Input: dimensioned drawing with shaded views. Units: mm. Origin: part minimum x, y, z. A direction names the side the tool comes from. Give positions to 0.01 mm unless a question says otherwise; leave off trailing zeros. Write each loop counter-clockwise with the first axis right and the second up, starting at its lowest first coordinate (ties: lowest second). Pieces come first, ordered by that corner, then holes.
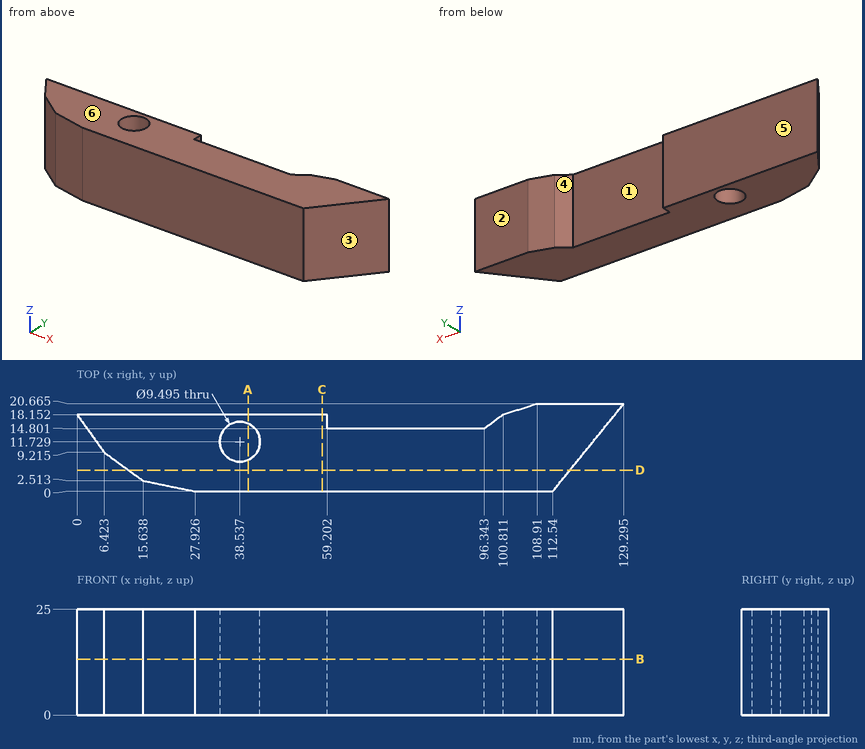
Item 1: Pull-direction query (X, two-part tool) for the marked faces 1, 2 and 3; classes: +X half, -X half, draft (parallel to the pull), parting line (faces both ways), or undercut.
Found:
face 1: undercut
face 2: draft
face 3: +X half
Item 2: Section D-D, the plane y = 5. Return the cut outline in (x, z), plus the area to 3 significant figures.
Found:
outline: (12.22, 0) - (116.59, 0) - (116.59, 25) - (12.22, 25) - close
area: 2,610 mm2
Item 3: Section B-B, the plane z = 13.25. Return the cut outline in (x, y) (1 decimal).
Found:
outline: (0, 18.2) - (6.4, 9.2) - (15.6, 2.5) - (27.9, 0) - (112.5, 0) - (129.3, 20.7) - (108.9, 20.7) - (100.8, 18.2) - (96.3, 14.8) - (59.2, 14.8) - (59.2, 18.2) - close; hole circle Ø9.5 at (38.5, 11.7)
Item 4: Section A-A, the plane x = 40.5. Return the cut outline in (y, z).
Found:
outline: (0, 0) - (7.41, 0) - (7.41, 25) - (0, 25) - close; (16.05, 0) - (18.15, 0) - (18.15, 25) - (16.05, 25) - close
Item 5: Reachability of the marked faces 4, 5 and 6 from +Z, -Z, +X, -X, +Y, -Y: full face, straight path, thin tool, end or side. Return the list, or none.
Found:
face 4: +Z, -Z, +Y
face 5: +Z, -Z, -X, +Y
face 6: +Z, +X, -X, +Y, -Y
Item 6: Section C-C, the plane x = 58. Return the cut outline in (y, z), plus the area to 3 significant figures.
Found:
outline: (0, 0) - (18.15, 0) - (18.15, 25) - (0, 25) - close
area: 454 mm2
Item 7: Pin query (flat end, axial travel): pin 1 Ø6 at (y, z) = (15, 3) entering from +X (1 decimal); pin 2 Ø3 at (x, z) = (15.5, 12.5) entering from +Y; pin 3 Ø7.5 at (x, z) = (85.5, 18) entering from +Y; pin 4 Ø7.5 at (x, y) = (38.54, 11.73) entering from +Z. Return the tip coordinate at first contact, or that it passes through.
Found:
pin 1: stops at x = 127.1
pin 2: stops at y = 18.15
pin 3: stops at y = 14.8
pin 4: passes through
Item 8: Line query: L1, parallel to Y at x = 39, z = 3.5 (1 decimal); L2, parallel to X at y = 8, z = 1 (1 decimal); L3, parallel to X at y = 16.75, z = 13 (1 decimal). Output: solid intervals per line, ascending.
Found:
L1: y = 0 to 7, 16.5 to 18.2
L2: x = 8.1 to 35.6, 41.5 to 119
L3: x = 1 to 59.2, 98.9 to 126.1
